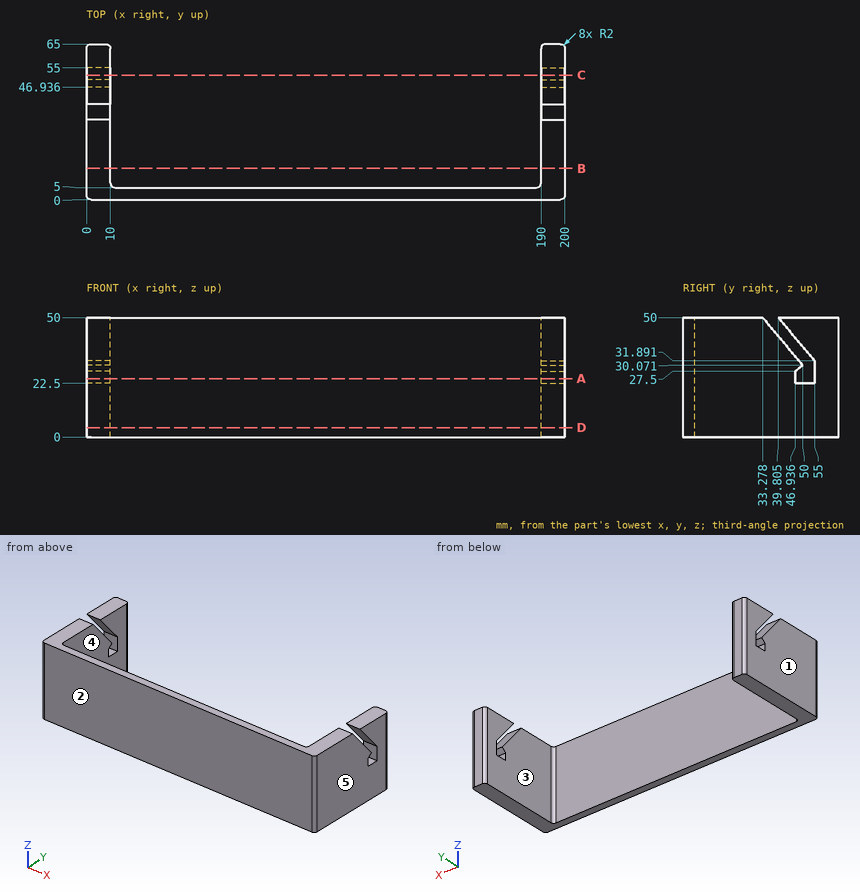
Here's the drawing with two shaded views (mm, measured from the low corner). I have some questions. A direction names the side the tool comes from. Round coordinates to 2 decimals unless told otherwise and drop trailing zeros. Order: outer loops, then holes, each group sorted by start corner. A loop starts at its lowest first (then second) coordinate and runs counter-clockwise, first axis right, second up. Notation, with made-up numbers: (-36, -22.5) -> (-28, -22.5) arc R28 ccw to (-28, -4.5) -> close; hole circle Ø5 at (74.25, 17.25). An arc over 180 degrees is marked (long way). Write each question's results on one line, items separated by ' | '. Start each with the question number.
Item 1: If we section it at B-B, the plane y = 13: Write out the boundary of the cut face in (x, z).
Item 2: If we section it at D-D, the plane z = 4: Write out the boundary of the cut face in (x, y).
Item 3: Please list where these lines run through material, in increasing order: L1, parallel to X at y = 15, z = 36.5; L2, parallel to Y at x = 40.5, z = 32; L3, parallel to X at y = 6, z = 19.
Item 4: Which directions (+Z, -Z, +X, -X, +Y, -Y) give clear straight access to the entire face, cutting with the end or side of a thin tool? Please do the marked faces 4 and 5.
Item 5: Thinking about a two-plate mould opening in X: for the marked faces 1, 2 and 3, which applies, +X half, -X half, draft (parallel to the pull), parting line (faces both ways), or undercut?
Item 6: If we section it at C-C, the plane y = 52: Write out the boundary of the cut face in (x, z).
Item 7: Will this pin go through, and if not, where does the flat tip stop? pin 1 (1 mm diameter, centred on x = 160, z = 40.5, fed in from +Y).
Item 8: If we section it at A-A, the plane z = 24.5: Write out the boundary of the cut face in (x, y).
Results:
1) outline: (0, 0) -> (10, 0) -> (10, 50) -> (0, 50) -> close; (190, 0) -> (200, 0) -> (200, 50) -> (190, 50) -> close
2) outline: (0, 2) arc R2 ccw to (2, 0) -> (198, 0) arc R2 ccw to (200, 2) -> (200, 63) arc R2 ccw to (198, 65) -> (192, 65) arc R2 ccw to (190, 63) -> (190, 7) arc R2 cw to (188, 5) -> (12, 5) arc R2 cw to (10, 7) -> (10, 63) arc R2 ccw to (8, 65) -> (2, 65) arc R2 ccw to (0, 63) -> close
3) L1: x = 0 to 10, 190 to 200 | L2: y = 0 to 5 | L3: x = 0 to 10.27, 189.73 to 200
4) face 4: +Z, -Z, +Y | face 5: +Z, -Z, +X, +Y, -Y
5) face 1: -X half | face 2: draft | face 3: undercut
6) outline: (0, 0) -> (10, 0) -> (10, 22.5) -> (0, 22.5) -> close; (0, 35.47) -> (10, 35.47) -> (10, 50) -> (0, 50) -> close; (190, 0) -> (200, 0) -> (200, 22.5) -> (190, 22.5) -> close; (190, 35.47) -> (200, 35.47) -> (200, 50) -> (190, 50) -> close
7) pin 1: stops at y = 5
8) outline: (0, 2) arc R2 ccw to (2, 0) -> (198, 0) arc R2 ccw to (200, 2) -> (200, 46.94) -> (190, 46.94) -> (190, 7) arc R2 cw to (188, 5) -> (12, 5) arc R2 cw to (10, 7) -> (10, 46.94) -> (0, 46.94) -> close; (0, 55) -> (10, 55) -> (10, 63) arc R2 ccw to (8, 65) -> (2, 65) arc R2 ccw to (0, 63) -> close; (190, 55) -> (200, 55) -> (200, 63) arc R2 ccw to (198, 65) -> (192, 65) arc R2 ccw to (190, 63) -> close
